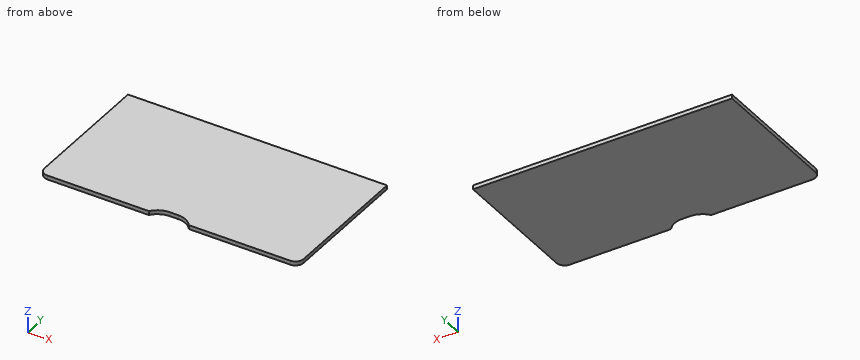
```python
from build123d import *

# Parameters (mm, degrees)
F0_W        = 64.5
F0_H        = 35
F1_DEPTH    = 1
F2_R        = 2
F3_W        = 10
F3_H        = 1
F4_DEPTH    = 2
F5_T1_DEPTH = 1


# Not quite as in the source:
# - a fillet or chamfer that OpenCascade refuses, or shapes differently, is made with other operations: its cross-section is extruded or revolved along the edge and cut away or added


with BuildPart() as f1:
    # F0 (on Top) → F1 (new body)
    with BuildSketch(Plane.XY):
        with Locations((0, -0.7672849298)):
            Rectangle(F0_W, F0_H)
    extrude(amount=F1_DEPTH)

    # F2
    f2_edges = [f1.edges().sort_by_distance(p)[0] for p in [
        (-32.25, -18.267285, 0.5),
        (32.25, -18.267285, 0.5),
    ]]
    fillet(f2_edges, radius=F2_R)

    # F3 (on face) → F4 (cut)
    with BuildSketch(Plane.XZ.offset(18.2672849298)):
        with Locations((0, 0.5)):
            Rectangle(F3_W, F3_H)
    extrude(amount=-F4_DEPTH, mode=Mode.SUBTRACT)

    # F5: fillet of radius 5 on 2 edges, made by hand

    # F5_s2 → F5_t1 (join)
    with BuildSketch(Plane.XY):
        with BuildLine():
            ThreePointArc((5, -18.2672849298), (3.2360679775, -16.7951489748), (1, -16.2672849298))
            Line((1, -16.2672849298), (5, -16.2672849298))
            Line((5, -16.2672849298), (5, -18.2672849298))
        make_face()
        with BuildLine():
            ThreePointArc((-1, -16.2672849298), (-3.2360679775, -16.7951489748), (-5, -18.2672849298))
            Line((-5, -18.2672849298), (-5, -16.2672849298))
            Line((-5, -16.2672849298), (-1, -16.2672849298))
        make_face()
    extrude(amount=F5_T1_DEPTH)


solid = f1.part
```
Build history of the part. All positions in model axes, mm. Give positions to 0.01 mm unless a question says otherwise; leave off trailing zeros. Loops run counter-clockwise (first coordinate to the right, second up) from the corner with the lowest first, then second, coordinate; pieces in that order, holes last.
1) Band-saw the part on A-A on x = 3. List the corners of the cut face in (y, z), then the cut area to 3 significant figures.
Values follow:
outline: (-16.68, 0) - (16.73, 0) - (16.73, 1) - (-16.68, 1) - close
area: 33.4 mm2
2) Drop a flat-ended pin along its axis: P1, Ø0.5, axis at x = 0.5, z = 0.5, coming from the -Y side. Give the stop position or say it passes through.
Values follow:
P1: stops at y = -16.27
3) Probe line 1 along Y through (x, z) = (-1, 0.1); line 2 along Y through (x, z) = (2.5, 0.5). List the from-to ranges inside material, lowest first.
Values follow:
line 1: y = -16.27 to 16.73
line 2: y = -16.5 to 16.73
